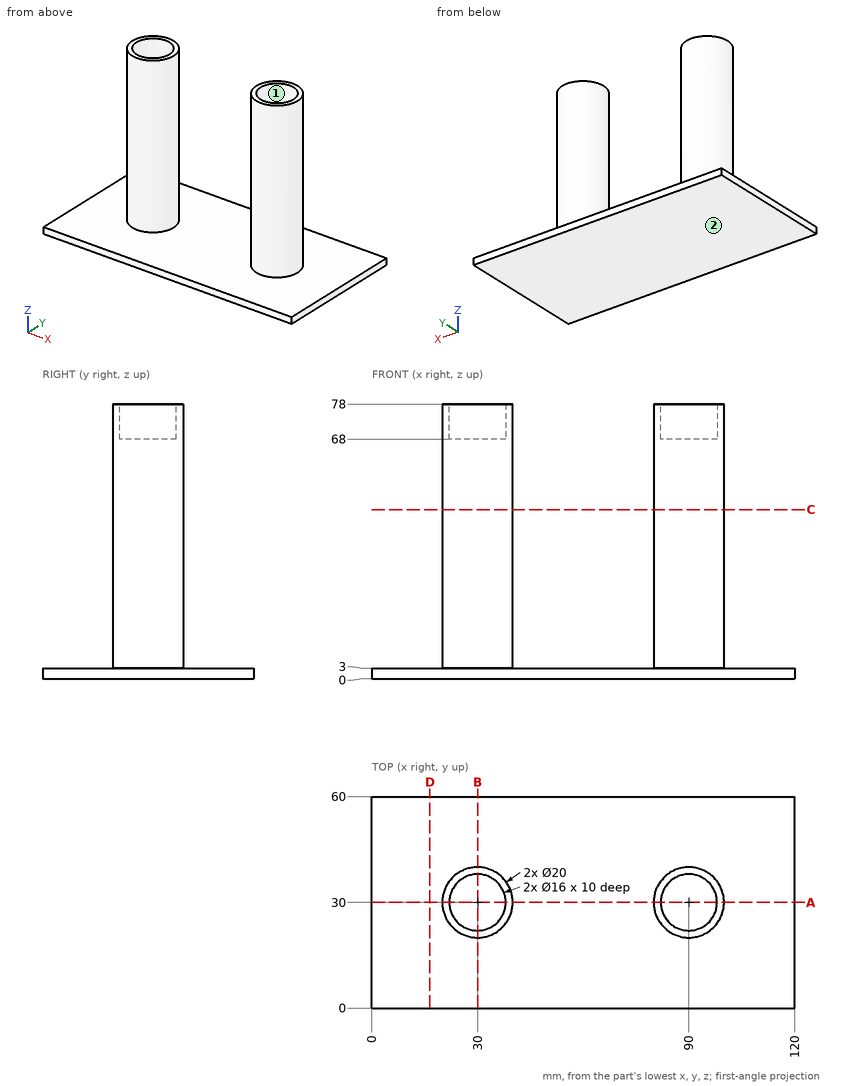
Input: dimensioned drawing with shaded views. Units: mm. Origin: part minimum x, y, z. Coordinates: 2 decimals unless noted, no trailing zeros. Order: outer loops, then holes, each group sorted by start corner. A loop starts at its lowest first (then second) coordinate and runs counter-clockwise, first axis right, second up.
(1) Section query C-C (z = 48). Return the cut outline in (x, y).
(2) Draft query along X for the marked faces 1 and 2. Return one class per face: pulls with the +X half, pulls with the -X half, needs draft (parallel to the pull), parting line crosses it, or undercut.
(3) First-contact query: pin 1 (13 mm diameter, centred on x = 33.5, y = 27.5, fed in from +Z); pin 2 (10 mm diameter, centred on x = 36.5, y = 14.5, fed in from +Z); pin 3 (8 mm diameter, centred on y = 45, z = 13.5, fed in from -X); pin 4 (14.5 mm diameter, centred on x = 90, y = 30, fed in from +Z). Flat tips, straight axial feed; report the tip coordinate or a pass-through.
(4) Section query B-B (x = 30). Return the cut outline in (y, z).
(5) Section query D-D (x = 16.5). Return the cut outline in (y, z), plus the area to 3 significant figures.
(6) Section query A-A (y = 30). Return the cut outline in (x, z), plus the area to 3 significant figures.
(7) Material intervals for probe 1 along X at (y, z) = (30.5, 73); probe 2 along Y at (x, z) = (90, 74); probe 3 along Z at (x, y) = (41.5, 22.5), sorted ascending.
Solution:
1. outline: circle Ø20 at (30, 30); circle Ø20 at (90, 30)
2. face 1: undercut
2. face 2: needs draft
3. pin 1: stops at z = 78
3. pin 2: stops at z = 3
3. pin 3: passes through
3. pin 4: stops at z = 68
4. outline: (0, 0) - (60, 0) - (60, 3) - (40, 3) - (40, 78) - (38, 78) - (38, 68) - (22, 68) - (22, 78) - (20, 78) - (20, 3) - (0, 3) - close
5. outline: (0, 0) - (60, 0) - (60, 3) - (0, 3) - close
5. area: 180 mm2
6. outline: (0, 0) - (120, 0) - (120, 3) - (100, 3) - (100, 78) - (98, 78) - (98, 68) - (82, 68) - (82, 78) - (80, 78) - (80, 3) - (40, 3) - (40, 78) - (38, 78) - (38, 68) - (22, 68) - (22, 78) - (20, 78) - (20, 3) - (0, 3) - close
6. area: 3,040 mm2
7. probe 1: x = 20.01 to 22.02, 37.98 to 39.99, 80.01 to 82.02, 97.98 to 99.99
7. probe 2: y = 20 to 22, 38 to 40
7. probe 3: z = 0 to 3
